Verification items for this drawing (mm, ordinates from the low corner). Give positions to 0.01 mm unless a question says otherwise; leave off trailing zeros. Order: outer loops, then holes, each group sorted by start corner. A loop starts at its lowest first (then second) coordinate and runs counter-clockwise, first axis right, second up. Notation, with made-up numbers: M 45,-23.5 L 54,-23.5 A21 ccw 54,10.5 Z; hole C 13,-29 d1. An arc over 180 degrees is marked long. Answer as a JSON object with one key per item and string values.
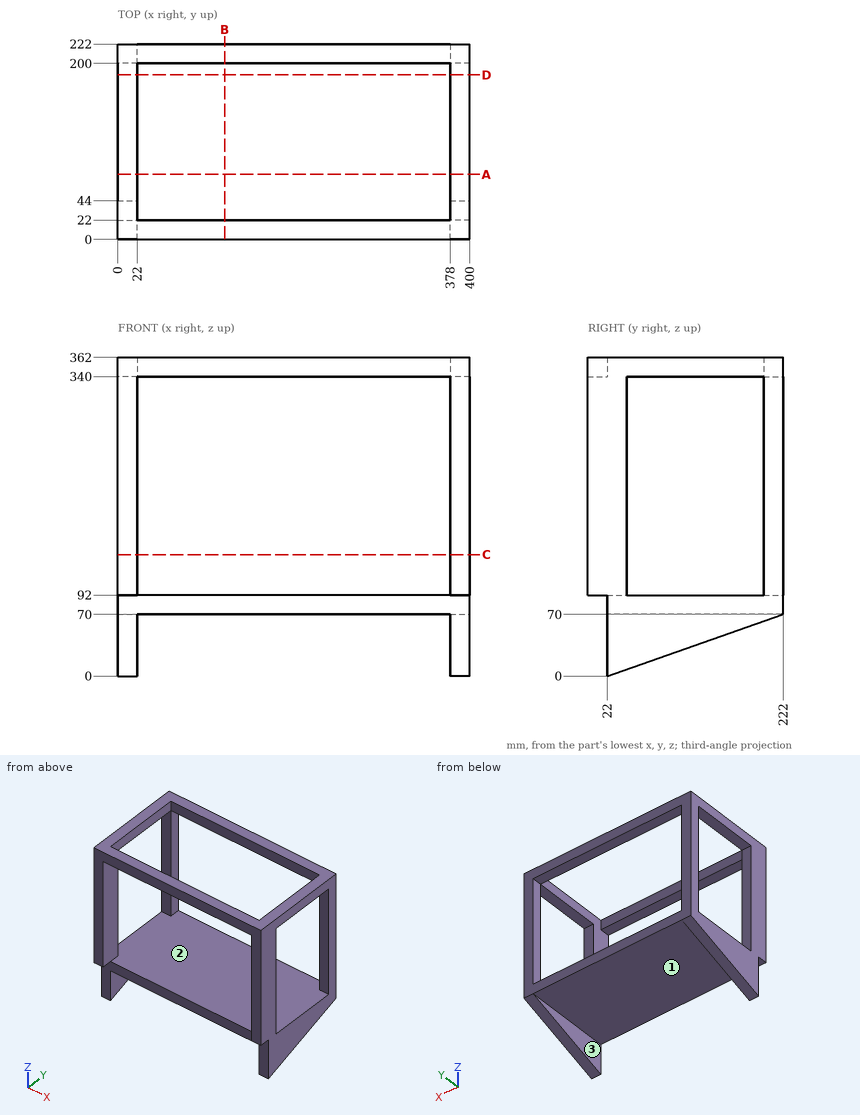
Q1. Section check C-C on z = 138. Record the cut outline in (x, y).
Resolved:
{"outline": "M 0,0 L 22,0 L 22,44 L 0,44 Z; M 0,200 L 22,200 L 22,222 L 0,222 Z; M 378,0 L 400,0 L 400,44 L 378,44 Z; M 378,200 L 400,200 L 400,222 L 378,222 Z"}
Q2. Gauge pin test, flat ends, axial feed: pin 1 Ø4 at (x, y) = (291.5, 104.5) entering from +Z; pin 2 Ø8 at (x, y) = (345.5, 116) entering from -Z; pin 3 Ø17.5 at (x, y) = (15.5, 92.5) entering from -Z. Record the tip position at first contact, or that the pin passes through.
Resolved:
{"pin 1": "stops at z = 92", "pin 2": "stops at z = 70", "pin 3": "stops at z = 21.61"}
Q3. Section check B-B on x = 121.5. Record the cut outline in (y, z), then the cut area to 3 significant figures.
Resolved:
{"outline": "M 0,340 L 22,340 L 22,362 L 0,362 Z; M 22,70 L 222,70 L 222,92 L 22,92 Z; M 200,340 L 222,340 L 222,362 L 200,362 Z", "area": "5,370 mm²"}
Q4. Release check for a two-part mould opening along Z. For the marked faces 1, 2 and 3 record: +Z half, -Z half, draft (parallel to the pull), parting line (faces both ways), or undercut.
Resolved:
{"face 1": "-Z half", "face 2": "undercut", "face 3": "draft"}
Q5. Section check A-A on y = 74. Record the cut outline in (x, z), then the cut area to 3 significant figures.
Resolved:
{"outline": "M 0,18.2 L 22,18.2 L 22,70 L 378,70 L 378,18.2 L 400,18.2 L 400,92 L 0,92 Z; M 0,340 L 22,340 L 22,362 L 0,362 Z; M 378,340 L 400,340 L 400,362 L 378,362 Z", "area": "12,000 mm²"}
Q6. Section check D-D on y = 187. Record the cut outline in (x, z), then the cut area to 3 significant figures.
Resolved:
{"outline": "M 0,57.75 L 22,57.75 L 22,70 L 378,70 L 378,57.75 L 400,57.75 L 400,92 L 0,92 Z; M 0,340 L 22,340 L 22,362 L 0,362 Z; M 378,340 L 400,340 L 400,362 L 378,362 Z", "area": "10,300 mm²"}
Q7. Material ranges on L1, parallel to Z at x = 343, y = 213.5; L2, parallel to X at y = 127, z = 68; L3, parallel to Z at x = 202, y = 70.5, recorded low to high.
Resolved:
{"L1": "z = 70 to 92, 340 to 362", "L2": "x = 0 to 22, 378 to 400", "L3": "z = 70 to 92"}
